Source: CAD feature listing. Evaluate the final solid. Frame: model axes, mm. Face numbers are marked on the shaded views. A direction names the side the tool comes from. Round coordinates to 2 decimals unless told otherwise and drop trailing zeros. Write each loop counter-clockwise with the first axis right and the second up, starting at its lowest first coordinate (ties: lowest second). Pieces come first, ordered by that corner, then holes. Notation, with made-up numbers: M -27.75,31 L 24.25,31 A18 cw 24.25,46 Z; hole C -17.5,77.25 d9. An arc over 180 degrees is marked long. Answer in a Markdown table with one row per item. Add a question column.
Item 1: Cut plane B-B on y = 0. Return loops of the section in (x, z), and give its area (3 significant figures).
Item 2: Contact query for flat-ended pins moving along their axis: pin 1 (5 mm diameter, centred on y = -11, z = 2.5, fed in from -X); pin 2 (12 mm diameter, centred on x = 16, y = 9.5, fed in from +Z); pin 3 (2 mm diameter, centred on y = -9.5, z = 7.5, fed in from +X). Output: stop coordinate, or through.
Item 3: Material intervals for probe 1 along Y at (x, z) = (46.5, 7.5); probe 2 along X at (y, z) = (0.5, 0.75); probe 3 along X at (y, z) = (6.5, 7), sorted ascending.
Item 4: Cut plane C-C on z = 2. Return loops of the section in (x, y).
Item 5: Cut plane A-A on x = 29. Return loops of the section in (y, z), and give its area (3 significant figures).
Item 6: Mould query, pull axis Y, two halves, no side actions, for the marked faces 3, 4 and 5. Classes: released by +Y, released by -Y, zero draft, split by the parting line, or undercut.
Item 7: Set-up query: the marked faces 1 and 2. Return all of +Z, -Z, +X, -X, +Y, -Y with unobstructed straight access to the full face (end or side cutting, diameter ignored); none if empty.
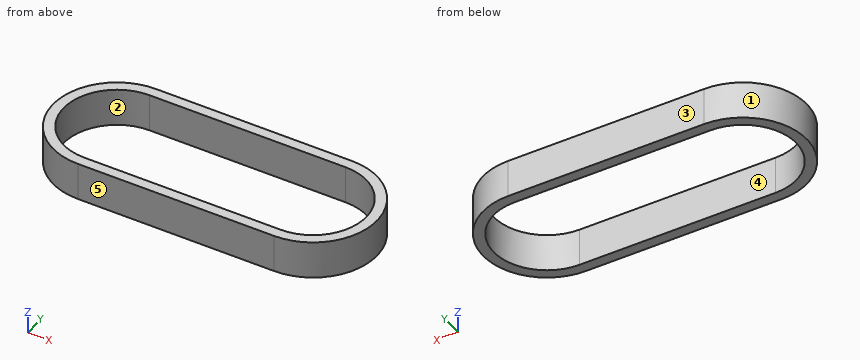
Autodesk Inventor part; units mm, degrees
ref_plane "YZ Plane" through (0, 0, 0) normal (1, 0, 0) x (0, 1, 0)
ref_plane "XZ Plane" through (0, 0, 0) normal (0, 1, 0) x (-1, 0, 0)
ref_plane "XY Plane" through (0, 0, 0) normal (0, 0, 1) x (1, 0, 0)
sketch "Sketch1" plane through (0, 0, 0) normal (0, 0, 1) x (1, 0, 0)
  arc A0 (0, 12.7381) -> (0, -12.7381) centre (0, 0) ccw
  arc A1 (47.498, -12.7381) -> (47.498, 12.7381) centre (47.498, 0) ccw
  line L0 (0, 12.7381) -> (47.498, 12.7381)
  line L1 (0, -12.7381) -> (47.498, -12.7381)
  line L2 (47.498, 15.2781) -> (0, 15.2781)
  arc A2 (0, 15.2781) -> (0, -15.2781) centre (0, 0) ccw
  line L3 (0, -15.2781) -> (47.498, -15.2781)
  arc A3 (47.498, -15.2781) -> (47.498, 15.2781) centre (47.498, 0) ccw
  dimension "d0" = 25.4762
  dimension "d1" = 47.498
  dimension "d2" = 2.54
extrude "Extrusion1" add sketch "Sketch1" along normal blind 9
properties part number "INDX_020_MiniFeederBelt" material "Rubber"
Results below:
| question | item | result |
|---|---|---|
| 1 | outline | M -15.28,0 L -12.74,0 L -12.74,9 L -15.28,9 Z; M 60.24,0 L 62.78,0 L 62.78,9 L 60.24,9 Z |
| 1 | area | 45.7 mm2 |
| 2 | pin 1 | x = -12.7 |
| 2 | pin 2 | z = 9 |
| 2 | pin 3 | x = 60.19 |
| 3 | probe 1 | -15.28 to -12.74, 12.74 to 15.28 |
| 3 | probe 2 | -15.27 to -12.73, 60.23 to 62.77 |
| 3 | probe 3 | -13.83 to -10.95, 58.45 to 61.32 |
| 4 | outline | M 0,-15.28 L 47.5,-15.28 A15.28 ccw 47.5,15.28 L 0,15.28 A15.28 ccw Z; hole M 0,-12.74 L 47.5,-12.74 A12.74 ccw 47.5,12.74 L 0,12.74 A12.74 ccw Z |
| 5 | outline | M -15.28,0 L -12.74,0 L -12.74,9 L -15.28,9 Z; M 12.74,0 L 15.28,0 L 15.28,9 L 12.74,9 Z |
| 5 | area | 45.7 mm2 |
| 6 | face 3 | released by +Y |
| 6 | face 4 | undercut |
| 6 | face 5 | released by -Y |
| 7 | face 1 | +Z, -Z, -X |
| 7 | face 2 | +Z, -Z |
